from build123d import *

# Parameters (mm, degrees)
BOSS_EXTRUDE1_DEPTH = 12


with BuildPart() as part:
    # Sketch1 → Boss-Extrude1 (new body)
    with BuildSketch(Plane.XY):
        Polygon((23.002215311, -29.371596289), (18.32005302, -25.71349019), (17.806104696, -26.07336068), (12.290321363, -29.935553749), (12.290321363, -41.394710348), (19.091253879, -46.156774563), (23.002215311, -43.055211302), align=None)
        Polygon((18.150250558, -26.564851907), (12.890321363, -30.24789398), (12.890321363, -41.082370118), (19.06894702, -45.408690378), (22.402215311, -42.765263014), (22.402215311, -29.664235842), (18.300514505, -26.459635958), align=None, mode=Mode.SUBTRACT)
    extrude(amount=BOSS_EXTRUDE1_DEPTH)


solid = part.part
The model under review builds one solid part; all positions refer to its coordinate system, in mm. A direction names the side the tool comes from. Round coordinates to 2 decimals unless told otherwise and drop trailing zeros. Write each loop counter-clockwise with the first axis right and the second up, starting at its lowest first coordinate (ties: lowest second). Pieces come first, ordered by that corner, then holes. Notation, with made-up numbers: (70.25, 33.25) - (107.25, 33.25) arc R15 cw to (107.25, 52.25) - close; hole circle Ø4 at (13, -10). An arc over 180 degrees is marked (long way). One line per item, written item: value. Start each with the question number.
1. Machinability: for faces 4 (the face through (23.002, -36, 6)), 5 (the face through (22.402, -36, 6)), which of the approach directions +Z, -Z, +X, -X, +Y, -Y give a long, thin tool a straight path to every point of the face, cutting with its end or side? Answer none if there is none.
2. The part is to be moulded in two halves that separate along Y. For faces 1 (the face through (21.019, -44.628, 5.916)), 2 (the face through (12.89, -36, 6)), 3 (the face through (12.5, -35.9, 0)), say which applies: released by +Y, released by -Y, zero draft, split by the parting line, or undercut.
3. Consider section A-A on y = -28. Write out the cut boundary in (x, z), and give its area (3 significant figures).
4. Consider section C-C on z = 9.75. Write out the cut boundary in (x, y), and give its area (3 significant figures).
5. To check wall thickness, follow L1, parallel to X at y = -34.75, z = 9; L2, parallel to X at y = -42.5, z = 7.25; L3, parallel to Y at x = 17.5, z = 5. State the ranges of each line that lie inside material, in increasing order. Write a range as from..to.
6. Clearance check with flat-ended pins moving along their axes: P1, Ø3, axis at x = 16, z = 2, coming from the -Y side; P2, Ø5, axis at x = 15, z = 3.5, coming from the +Y side. State where each tip first meets the part, or that it passes through.
7. Consider section B-B on x = 22. Write out the cut boundary in (y, z).
Checks:
1. face 4: +Z, -Z, +X, +Y, -Y
1. face 5: +Z, -Z
2. face 1: released by -Y
2. face 2: undercut
2. face 3: zero draft
3. outline: (15.05, 0) - (16.1, 0) - (16.1, 12) - (15.05, 12) - close; (20.27, 0) - (21.25, 0) - (21.25, 12) - (20.27, 12) - close
3. area: 24.2 mm^2
4. outline: (12.29, -41.39) - (19.09, -46.16) - (23, -43.06) - (23, -29.37) - (18.32, -25.71) - (12.29, -29.94) - close; hole (12.89, -41.08) - (19.07, -45.41) - (22.4, -42.77) - (22.4, -29.66) - (18.3, -26.46) - (12.89, -30.25) - close
4. area: 29.8 mm^2
5. L1: x = 12.29..12.89, 22.4..23
5. L2: x = 13.87..14.91, 22.4..23
5. L3: y = -45.04..-44.31, -27.02..-26.29
6. P1: stops at y = -45.04
6. P2: stops at y = -26.29
7. outline: (-43.85, 0) - (-43.08, 0) - (-43.08, 12) - (-43.85, 12) - close; (-29.35, 0) - (-28.59, 0) - (-28.59, 12) - (-29.35, 12) - close
